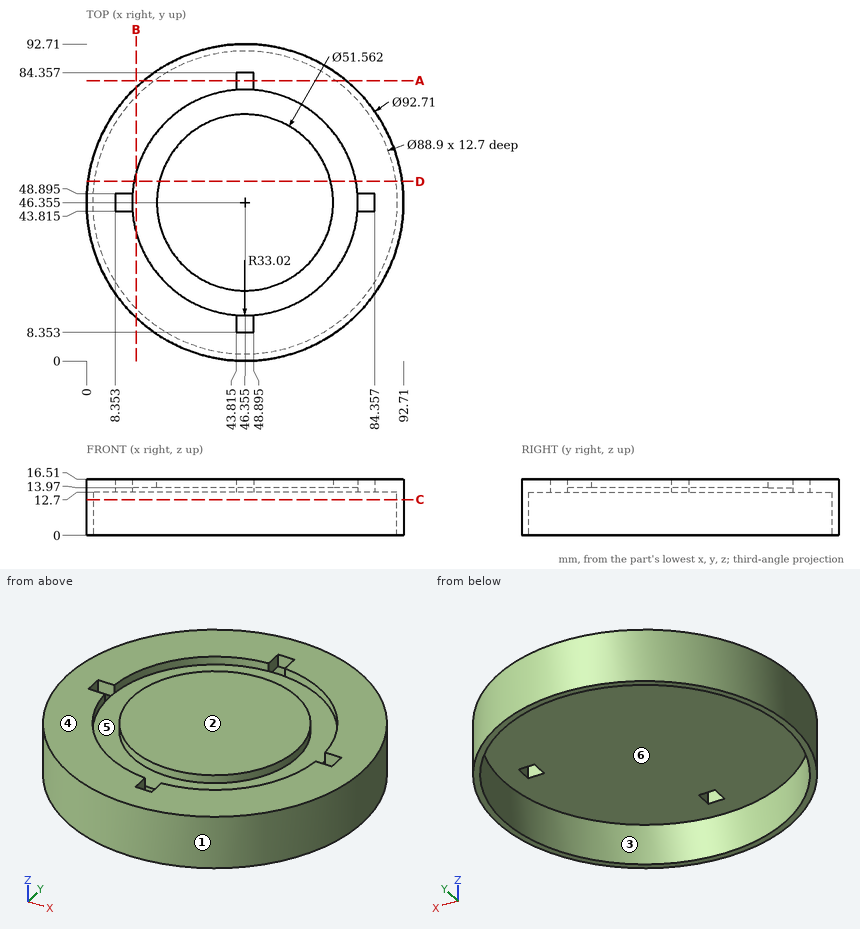
The figure shows three views and two pictorial views of one solid part (mm, origin at its lowest corner). Answer the questions. A direction names the side the tool comes from. Give positions to 0.01 mm unless a question says otherwise; leave off trailing zeros. Write each loop counter-clockwise with the first axis right and the second up, starting at its lowest first coordinate (ties: lowest second). Pieces come first, ordered by that corner, then holes. Notation, with made-up numbers: M 81,64.25 L 93,64.25 A17 cw 93,77.25 Z; hole C -33,58.25 d11. An arc over 180 degrees is marked long. One line per item, written item: value. Start each with the question number.
(1) Find section D-D (y = 52.5). Determine the outline of the cut face in (x, z), plus the area to 3 significant figures.
(2) Find section A-A (y = 82). Determine the outline of the cut face in (x, z) (1 decimal), plus the area to 3 significant figures.
(3) Determine the mould class of the marked faces 1, 2 and 3 for opening direction Y: pulls with the +Y half, pulls with the -Y half, needs draft (parallel to the pull), parting line crosses it, or undercut.
(4) Flat-ended cylindrical pins translate along their axes: pin 1 Ø4 at (x, z) = (82.5, 14.5) entering from -Y; pin 2 Ø4 at (y, z) = (9.5, 7.5) entering from +X (1 decimal); pin 3 Ø8 at (x, z) = (36, 12.5) entering from -Y. Find the tip coordinate at first contact, or state that the pin passes through.
(5) Find section B-B (x = 14.5). Determine the outline of the cut face in (y, z), plus the area to 3 significant figures.
(6) A tool of negligible diameter and unlimited length cuts with its end or side. For the marked faces 4, 5 and 6, from which of +Z, -Z, +X, -X, +Y, -Y can it reach the whole face along a straight path? Write none if from no direction.
(7) Find the intervals of material crossed by line 1 (Y direction, x = 47, z = 14.5); line 2 (Y direction, x = 70, z = 15.25) (1 decimal); line 3 (Z direction, x = 51.5, y = 27), in increasing order.
(8) Find section C-C (z = 10.5). Determine the outline of the cut face in (x, y) (3 decimals).
Results below:
1. outline: M 0.41,0 L 2.33,0 L 2.33,12.7 L 90.38,12.7 L 90.38,0 L 92.3,0 L 92.3,16.51 L 78.8,16.51 L 78.8,13.97 L 71.39,13.97 L 71.39,16.51 L 21.32,16.51 L 21.32,13.97 L 13.91,13.97 L 13.91,16.51 L 0.41,16.51 Z
1. area: 361 mm^2
2. outline: M 16.7,0 L 19.8,0 L 19.8,12.7 L 43.8,12.7 L 43.8,16.5 L 16.7,16.5 Z; M 48.9,12.7 L 72.9,12.7 L 72.9,0 L 76,0 L 76,16.5 L 48.9,16.5 Z
2. area: 285 mm^2
3. face 1: parting line crosses it
3. face 2: needs draft
3. face 3: undercut
4. pin 1: stops at y = 15
4. pin 2: stops at x = 76.9
4. pin 3: stops at y = 0.44
5. outline: M 12.68,0 L 15.35,0 L 15.35,12.7 L 77.36,12.7 L 77.36,0 L 80.03,0 L 80.03,16.51 L 55.05,16.51 L 55.05,13.97 L 37.66,13.97 L 37.66,16.51 L 12.68,16.51 Z
5. area: 280 mm^2
6. face 4: +Z, +X, -X, +Y, -Y
6. face 5: +Z
6. face 6: -Z
7. line 1: y = 0 to 8.35, 20.58 to 72.13, 84.36 to 92.71
7. line 2: y = 6.5 to 23.3, 36.1 to 56.6, 69.4 to 86.2
7. line 3: z = 12.7 to 16.51
8. outline: C 46.355,46.355 d92.71; hole C 46.355,46.355 d88.9
